from build123d import *

# Parameters (mm, degrees)
F0_W     = 19.05
F0_H     = 19.05
F3_W     = 19.05
F3_H     = 19.05
F4_DEPTH = 904.875


with BuildPart() as f2:
    # F2: sweep along a path in F1
    with BuildLine(Plane.XY) as f2_path:
        Line((914.4, -304.8), (-914.4, -304.8))
        Line((-914.4, -304.8), (-914.4, 304.8))
        Line((-914.4, 304.8), (914.4, 304.8))
        Line((914.4, 304.8), (914.4, -304.8))
    # F0 (on Right) → F2 (sweep)
    with BuildSketch(Plane.YZ):
        with BuildLine():
            Line((-282.575, 12.7), (-301.625, 12.7))
            ThreePointArc((-301.625, 12.7), (-303.8700640303, 11.7700640303), (-304.8, 9.525))
            Line((-304.8, 9.525), (-304.8, -9.525))
            ThreePointArc((-304.8, -9.525), (-303.8700640303, -11.7700640303), (-301.625, -12.7))
            Line((-301.625, -12.7), (-282.575, -12.7))
            ThreePointArc((-282.575, -12.7), (-280.3299359697, -11.7700640303), (-279.4, -9.525))
            Line((-279.4, -9.525), (-279.4, 9.525))
            ThreePointArc((-279.4, 9.525), (-280.3299359697, 11.7700640303), (-282.575, 12.7))
        make_face()
        with Locations((-292.1, 0)):
            Rectangle(F0_W, F0_H, mode=Mode.SUBTRACT)
    sweep(path=f2_path.line, transition=Transition.RIGHT)

    # F3 (on Right) → F4 (join, symmetric)
    with BuildSketch(Plane.YZ):
        with BuildLine():
            Line((-180.975, 12.7), (-200.025, 12.7))
            ThreePointArc((-200.025, 12.7), (-202.2700640303, 11.7700640303), (-203.2, 9.525))
            Line((-203.2, 9.525), (-203.2, -9.525))
            ThreePointArc((-203.2, -9.525), (-202.2700640303, -11.7700640303), (-200.025, -12.7))
            Line((-200.025, -12.7), (-180.975, -12.7))
            ThreePointArc((-180.975, -12.7), (-178.7299359697, -11.7700640303), (-177.8, -9.525))
            Line((-177.8, -9.525), (-177.8, 9.525))
            ThreePointArc((-177.8, 9.525), (-178.7299359697, 11.7700640303), (-180.975, 12.7))
        make_face()
        with Locations((-190.5, 0)):
            Rectangle(F3_W, F3_H, mode=Mode.SUBTRACT)
        with BuildLine():
            ThreePointArc((200.025, -12.7), (202.2700640303, -11.7700640303), (203.2, -9.525))
            Line((203.2, -9.525), (203.2, 9.525))
            ThreePointArc((203.2, 9.525), (202.2700640303, 11.7700640303), (200.025, 12.7))
            Line((200.025, 12.7), (180.975, 12.7))
            ThreePointArc((180.975, 12.7), (178.7299359697, 11.7700640303), (177.8, 9.525))
            Line((177.8, 9.525), (177.8, -9.525))
            ThreePointArc((177.8, -9.525), (178.7299359697, -11.7700640303), (180.975, -12.7))
            Line((180.975, -12.7), (200.025, -12.7))
        make_face()
        with Locations((190.5, 0)):
            Rectangle(F3_W, F3_H, mode=Mode.SUBTRACT)
    extrude(amount=F4_DEPTH, both=True)


solid = f2.part
Geometry: final body of the model. Coordinates: model frame, mm. A direction names the side the tool comes from. Give positions to 0.01 mm unless a question says otherwise; leave off trailing zeros. Write each loop counter-clockwise with the first axis right and the second up, starting at its lowest first coordinate (ties: lowest second). Pieces come first, ordered by that corner, then holes. Notation, with made-up numbers: (55, -37) -> (59, -37) arc R16 ccw to (59, -12) -> close; hole circle Ø9 at (-32, 68.5). An arc over 180 degrees is marked (long way). Answer in a Markdown table with one row per item.
(1) Draft query along X for faces 3 (the flat face through (-4.3, -199.7, 12.7)), 4 (the flat face through (-4, -289, -9.525)). Return one class per face: +X half, -X half, draft (parallel to the pull), parting line (faces both ways), or undercut.
Answers below:
| item | result |
|---|---|
| face 3 | draft |
| face 4 | undercut |
(2) Set-up query: faces 1 (the flat face through (-4, 289, 9.525)), 2 (the flat face through (4.3, 199.7, -12.7)). Return all of +Z, -Z, +X, -X, +Y, -Y with unobstructed straight access to the full face (end or side cutting, diameter ignored); none if empty.
Answers below:
| item | result |
|---|---|
| face 1 | none |
| face 2 | -Z, +X, -X, +Y, -Y |
(3) Section query A-A on y = 76. Return loops of the section in (x, z) (3 decimals), then the cut area to 3 significant figures.
Answers below:
| item | result |
|---|---|
| outline | (-914.4, -9.525) arc R3.175 ccw to (-911.225, -12.7) -> (-892.175, -12.7) arc R3.175 ccw to (-889, -9.525) -> (-889, 9.525) arc R3.175 ccw to (-892.175, 12.7) -> (-911.225, 12.7) arc R3.175 ccw to (-914.4, 9.525) -> close; (889, -9.525) arc R3.175 ccw to (892.175, -12.7) -> (911.225, -12.7) arc R3.175 ccw to (914.4, -9.525) -> (914.4, 9.525) arc R3.175 ccw to (911.225, 12.7) -> (892.175, 12.7) arc R3.175 ccw to (889, 9.525) -> close; hole (-911.225, -9.525) -> (-892.175, -9.525) -> (-892.175, 9.525) -> (-911.225, 9.525) -> close; hole (892.175, -9.525) -> (911.225, -9.525) -> (911.225, 9.525) -> (892.175, 9.525) -> close |
| area | 547 mm^2 |
(4) Ray query, line 1 along X through (y, z) = (-44, 5) (3 decimals); line 2 along Y through (x, z) = (794.5, 9.75); line 3 along X through (y, z) = (-148.5, 10.75). Return the intervals inside material, ascending. Write a range as [from, to].
Answers below:
| item | result |
|---|---|
| line 1 | [-914.4, -911.225], [-892.175, -889], [889, 892.175], [911.225, 914.4] |
| line 2 | [-304.79, -279.41], [-203.19, -177.81], [177.81, 203.19], [279.41, 304.79] |
| line 3 | [-914.15, -889.25], [889.25, 914.15] |
(5) Section query B-B on z = 3. State how many separate pieces and enclosed holes the cut face has, then the cut area to 3 significant figures.
Answers below:
| item | result |
|---|---|
| separate pieces | 2 |
| enclosed holes | 6 |
| area | 53,200 mm^2 |
